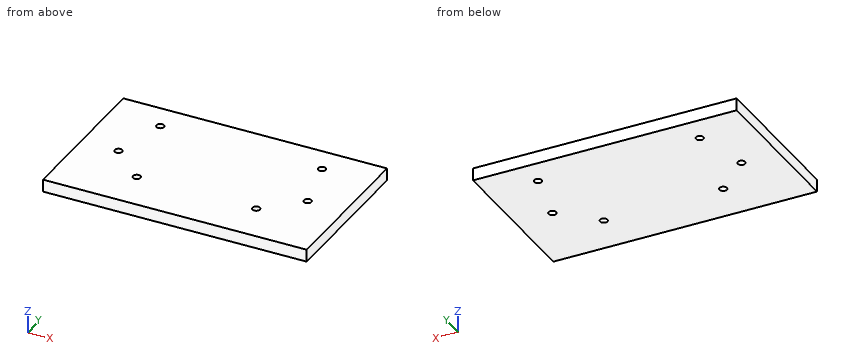
```python
from build123d import *

# Parameters (mm, degrees)
SKETCH1_W           = 106
SKETCH1_H           = 63
BOSS_EXTRUDE1_DEPTH = 5
SKETCH2_R           = 1.5
CUT_EXTRUDE2_DEPTH  = 6


with BuildPart() as part:
    # Sketch1 → Boss-Extrude1 (new body)
    with BuildSketch(Plane.XY):
        Rectangle(SKETCH1_W, SKETCH1_H)
    extrude(amount=BOSS_EXTRUDE1_DEPTH)

    # Sketch2 → Cut-Extrude2 (cut, through all)
    with BuildSketch(Plane.XY):
        with Locations((-24, -14.5)):
            Circle(SKETCH2_R)
        with Locations((24, -14.5)):
            Circle(SKETCH2_R)
        with Locations((-38, -1.5)):
            Circle(SKETCH2_R)
        with Locations((38, -1.5)):
            Circle(SKETCH2_R)
        with Locations((-32.5, 20.5)):
            Circle(SKETCH2_R)
        with Locations((32.5, 20.5)):
            Circle(SKETCH2_R)
    extrude(amount=CUT_EXTRUDE2_DEPTH, mode=Mode.SUBTRACT)


solid = part.part
```
Can you work these out from the model? Positions are in its coordinate system, mm. Coordinates: 2 decimals unless noted, no trailing zeros. Loops run counter-clockwise (first coordinate to the right, second up) from the corner with the lowest first, then second, coordinate; pieces in that order, holes last. Notation, with made-up numbers: M 58,18.25 L 104,18.25 A18 ccw 104,47.25 Z; hole C -5,75.25 d8. An arc over 180 degrees is marked long. Put each result on its own line as item: value. Start each with the question number.
(1) Imagine slicing it at A-A on y = -14.5. List the corners of the cut face in (x, z) for me.
(2) I need wall thicknesses on probe 1 along X at (y, z) = (-14.5, 2.4); probe 2 along Y at (x, z) = (24, 2.35); probe 3 along Y at (x, z) = (32.5, 3.95). Which ranges of each line are inside material? Lowest first, please.
(3) Imagine slicing it at B-B on x = -38. List the corners of the cut face in (y, z) for me.
Worked answers:
1. outline: M -53,0 L -25.5,0 L -25.5,5 L -53,5 Z; M -22.5,0 L 22.5,0 L 22.5,5 L -22.5,5 Z; M 25.5,0 L 53,0 L 53,5 L 25.5,5 Z
2. probe 1: x = -53 to -25.5, -22.5 to 22.5, 25.5 to 53
2. probe 2: y = -31.5 to -16, -13 to 31.5
2. probe 3: y = -31.5 to 19, 22 to 31.5
3. outline: M -31.5,0 L -3,0 L -3,5 L -31.5,5 Z; M 0,0 L 31.5,0 L 31.5,5 L 0,5 Z
